Here's how the part is built. I have some questions about the finished solid (model axes, mm). A direction names the side the tool comes from. Round coordinates to 2 decimals unless told otherwise and drop trailing zeros. Loops run counter-clockwise (first coordinate to the right, second up) from the corner with the lowest first, then second, coordinate; pieces in that order, holes last. Notation, with made-up numbers: (14.25, -29.75) -> (62.25, -29.75) arc R37 ccw to (62.25, 9.25) -> close; hole circle Ø7 at (-10, 46.25). An arc over 180 degrees is marked (long way). Use one line per item in the form item = value. Start each with the question number.
Item 1: I'm going to push flat-ended pins straight in: pin 1 Ø12.5 at (y, z) = (-3.5, 4.5) entering from +X; pin 2 Ø10 at (y, z) = (-2.5, -6.5) entering from -X; pin 3 Ø8.5 at (y, z) = (-2.5, 6) entering from -X; pin 4 Ø4 at (x, z) = (7, 10.5) entering from +Y. Where does each tip first touch, or does it pass through?
Item 2: If we section it at A-A (x = 3.25): Write out the boundary of the cut face in (y, z).
Item 3: For faces 1 (the face through (4.51, -4.21, -13.35)), 2 (the face through (0.908, -0.66, 14.985)), 3 (the face through (4.796, -3.755, -11.923)), which set-ups out of +Z, -Z, +X, -X, +Y, -Y let a thin tool reach every point of the face, with its end or its side?
Item 4: Thinking about a two-plate mould opening in Z: for faces 4 (the face through (9, -13, 2)), 5 (the face through (1, -10.24, 1.91)), 6 (the face through (2.007, 5.554, -13.394)), 7 (the face through (0.756, 10.006, 2.222)), which applies, released by +Z, released by -Z, zero draft, split by the parting line, or undercut?
Item 5: If I drill on L1, parallel to Y at x = 0.7, z = 0; L2, parallel to X at y = 11.75, z = 4; L3, parallel to Y at x = 8.25, z = 7.5, over which ranges is the centre line in solid material (lowest first)? Write a range as [from, to].
```python
from build123d import *

# Parameters (mm, degrees)
THREAD2_PITCH = 1


with BuildPart() as part:
    # Sketch1 → Revolve1 (revolve)
    with BuildSketch(Plane.XY, mode=Mode.PRIVATE) as revolve1_sk:
        Polygon((0, -11.15), (0, -14.7), (0.3, -15), (1.5, -15), (1.5, -14.5), (2.5, -14.5), (2.5, -15), (4, -15), (4, -14), (5, -14), (5, -14.5), (8.7, -14.5), (9, -14.2), (9, -12.8), (8.7, -12.5), (1, -12.5), (1, -10.25), (0.519615242, -10.25), align=None)
    revolve(revolve1_sk.sketch.rotate(Axis((35.470277062, 0, 0), (-1, 0, 0)), 270), axis=Axis((35.470277062, 0, 0), (-1, 0, 0)))

    # Thread2: the profile of Thread Profile2 profile screwed along a right-hand helix of 4 turns, 8 arcs to a turn; built about Z, then put on its axis
    thread2_z = Axis((0, 0, 0), (0, 0, 1))
    thread2_corners = [(14.5003, 0, 0.750173208), (13.95873412, 0, 0.437500002), (13.95873412, 0, 0.312500002), (14.5003, 0, -0.000173205)]
    with BuildLine(mode=Mode.PRIVATE) as thread2_profile:
        Line(thread2_corners[0], thread2_corners[1])
        Line(thread2_corners[1], thread2_corners[2])
        Line(thread2_corners[2], thread2_corners[3])
        Line(thread2_corners[3], thread2_corners[0])
    thread2_cap = Face(thread2_profile.wire())
    thread2_turn_angles = [0, 22.5, 45, 67.5, 90, 112.5, 135, 157.5, 180, 202.5, 225, 247.5, 270, 292.5, 315, 337.5, 360]
    thread2_turn_weights = [1, 0.9238795325112867, 1, 0.9238795325112867, 1, 0.9238795325112867, 1, 0.9238795325112867, 1, 0.9238795325112867, 1, 0.9238795325112867, 1, 0.9238795325112867, 1, 0.9238795325112867, 1]
    thread2_turn_rails = [Edge.make_bspline([Vector(p[0], p[1], 0).rotate(thread2_z, thread2_turn_angles[k]) / thread2_turn_weights[k] + Vector(0, 0, p[2] + THREAD2_PITCH * thread2_turn_angles[k] / 360) for k in range(17)], [0, 0, 0, 1, 1, 2, 2, 3, 3, 4, 4, 5, 5, 6, 6, 7, 7, 8, 8, 8], 2, thread2_turn_weights) for p in thread2_corners]
    thread2_turn_sides = [Face.make_surface_from_curves(thread2_turn_rails[p[0]], thread2_turn_rails[p[1]]) for p in [(0, 1), (1, 2), (2, 3), (3, 0)]]
    thread2 = Plane(origin=(9, 0, 0), x_dir=(0, 1, 0), z_dir=(-1, 0, 0)) * Solid(Shell([*[p.moved(Location((0, 0, THREAD2_PITCH * i))) for i in range(4) for p in thread2_turn_sides], thread2_cap, thread2_cap.rotate(thread2_z, 1440).moved(Location((0, 0, THREAD2_PITCH * 1440 / 360)))]))
    add(thread2, mode=Mode.SUBTRACT)


solid = part.part
```
Values found:
q1.pin_1 = 1
q1.pin_2 = 0
q1.pin_3 = 0.23
q1.pin_4 = 11.75
q2.outline = circle Ø30 at (0, 0); hole circle Ø25 at (0, 0)
q3.face_1 = none
q3.face_2 = +X, -X
q3.face_3 = +X
q4.face_4 = zero draft
q4.face_5 = undercut
q4.face_6 = split by the parting line
q4.face_7 = undercut
q5.L1 = [-15, -10.25], [10.25, 15]
q5.L2 = [0, 1]
q5.L3 = [-12.08, -10], [10, 12.41]
